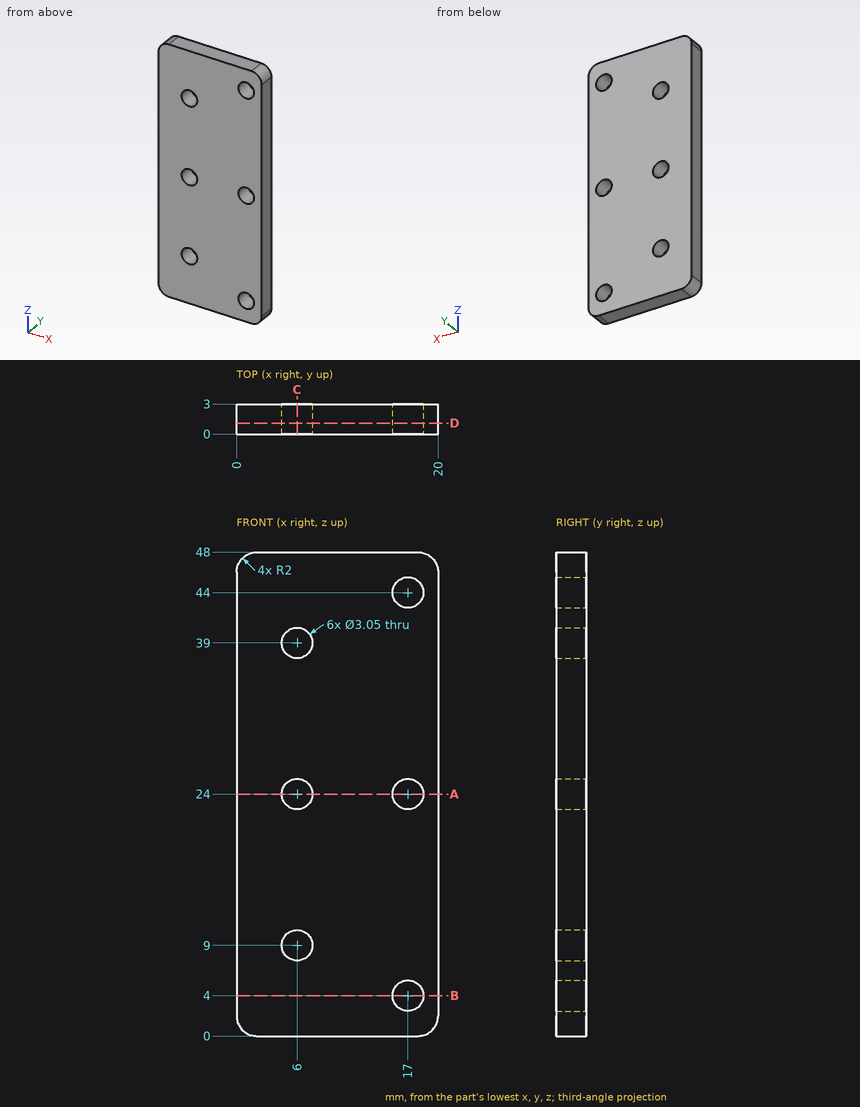
The drawing under review shows one solid part. Ordinate dimensions are in mm from its lowest x, y, z. Coordinates: 2 decimals unless noted, no trailing zeros. Loops run counter-clockwise (first coordinate to the right, second up) from the corner with the lowest first, then second, coordinate; pieces in that order, holes last. Notation, with made-up numbers: (38, 81) - (87, 81) arc R16 cw to (87, 90) - close; hole circle Ø11 at (29.25, 37.25). An arc over 180 degrees is marked (long way). Use CSV: the item, a comma, the result in double quotes. Start each with the question number.
1. Add section C-C on x = 6. Give the boundary of the cut face in (y, z) (3 decimals), plus the area to 3 significant figures.
2. Add section D-D on y = 1.1. Give the boundary of the cut face in (x, z) (3 decimals).
3. To check wall thickness, follow probe 1 along Z at (x, y) = (17, 2.4) (3 decimals); probe 2 along X at (y, z) = (2.2, 24) (3 decimals); probe 3 along Z at (x, y) = (6, 1.35) (3 decimals). State the ranges of each line that lie inside material, in increasing order.
4. Add section B-B on z = 4. Give the boundary of the cut face in (x, y) (3 decimals), plus the area to 4 significant figures.
5. Add section A-A on z = 24. Give the boundary of the cut face in (x, y) (3 decimals).
6. Clearance check with a flat-ended pin moving along its axis: pin 1 (1.8 mm diameter, centred on x = 17, z = 24, fed in from -Y). State where the tip first meets the part, or that it passes through.
Resolved:
1,outline,"(0, 0) - (3, 0) - (3, 7.475) - (0, 7.475) - close; (0, 10.525) - (3, 10.525) - (3, 22.475) - (0, 22.475) - close; (0, 25.525) - (3, 25.525) - (3, 37.475) - (0, 37.475) - close; (0, 40.525) - (3, 40.525) - (3, 48) - (0, 48) - close"
1,area,"117 mm2"
2,outline,"(0, 2) arc R2 ccw to (2, 0) - (18, 0) arc R2 ccw to (20, 2) - (20, 46) arc R2 ccw to (18, 48) - (2, 48) arc R2 ccw to (0, 46) - close; hole circle Ø3.05 at (6, 9); hole circle Ø3.05 at (6, 24); hole circle Ø3.05 at (6, 39); hole circle Ø3.05 at (17, 4); hole circle Ø3.05 at (17, 24); hole circle Ø3.05 at (17, 44)"
3,probe 1,"0 to 2.475, 5.525 to 22.475, 25.525 to 42.475, 45.525 to 48"
3,probe 2,"0 to 4.475, 7.525 to 15.475, 18.525 to 20"
3,probe 3,"0 to 7.475, 10.525 to 22.475, 25.525 to 37.475, 40.525 to 48"
4,outline,"(0, 0) - (15.475, 0) - (15.475, 3) - (0, 3) - close; (18.525, 0) - (20, 0) - (20, 3) - (18.525, 3) - close"
4,area,"50.85 mm2"
5,outline,"(0, 0) - (4.475, 0) - (4.475, 3) - (0, 3) - close; (7.525, 0) - (15.475, 0) - (15.475, 3) - (7.525, 3) - close; (18.525, 0) - (20, 0) - (20, 3) - (18.525, 3) - close"
6,pin 1,"through"
